from build123d import *

# Parameters (mm, degrees)
SKETCH1_W           = 39.4
SKETCH1_H           = 16.4
SKETCH1_R           = 1.725
BOSS_EXTRUDE1_DEPTH = 1.2
SKETCH2_W           = 12.5
SKETCH2_H           = 4
SKETCH2_W_2         = 4
SKETCH2_H_2         = 10.5
BOSS_EXTRUDE2_DEPTH = 2.5
SKETCH3_W           = 11.3
SKETCH3_H           = 12.5
SKETCH3_W_2         = 12.75
SKETCH3_H_2         = 6.6
BOSS_EXTRUDE3_DEPTH = 6
BOSS_EXTRUDE4_DEPTH = 2


with BuildPart() as part:
    # Sketch1 → Boss-Extrude1 (new body)
    with BuildSketch(Plane(origin=(0, 0, 0), x_dir=(1, 0, 0), z_dir=(0, 1, 0))):
        Rectangle(SKETCH1_W, SKETCH1_H)
        with Locations(Location((-16.7, 5.2, 0), (0, 0, 270))):
            Circle(SKETCH1_R, mode=Mode.SUBTRACT)
        with Locations(Location((2.3, 5.2, 0), (0, 0, 270))):
            Circle(SKETCH1_R, mode=Mode.SUBTRACT)
    extrude(amount=BOSS_EXTRUDE1_DEPTH)

    # Sketch2 → Boss-Extrude2 (add)
    with BuildSketch(Plane(origin=(0, 1.2, 0), x_dir=(1, 0, 0), z_dir=(0, 1, 0))):
        with Locations((-7.45, -1.2)):
            Rectangle(SKETCH2_W, SKETCH2_H)
        with Locations((8.2, -0.05)):
            Rectangle(SKETCH2_W_2, SKETCH2_H_2)
    extrude(amount=BOSS_EXTRUDE2_DEPTH)

    # Sketch3 → Boss-Extrude3 (add)
    with BuildSketch(Plane.XZ):
        with Locations((14.05, 0)):
            Rectangle(SKETCH3_W, SKETCH3_H)
        with Locations((-7.2, -4.9)):
            Rectangle(SKETCH3_W_2, SKETCH3_H_2)
    extrude(amount=BOSS_EXTRUDE3_DEPTH)

    # Sketch4 → Boss-Extrude4 (add, symmetric)
    with BuildSketch(Plane(origin=(0, -3, 0), x_dir=(-1, 0, 0), z_dir=(0, -1, 0))):
        with BuildLine():
            Line((1.825, 8.2), (13.224013115, 11.95))
            ThreePointArc((13.224013115, 11.95), (14.96605462, 13.598761551), (16.825, 12.083028945))
            Line((16.825, 12.083028945), (16.627742085, 12.050024171))
            ThreePointArc((16.627742085, 12.050024171), (14.909005352, 13.395228648), (13.416459603, 11.802765704))
            Line((13.416459603, 11.802765704), (2.465, 8.2))
            Line((2.465, 8.2), (1.825, 8.2))
        make_face()
    extrude(amount=BOSS_EXTRUDE4_DEPTH, both=True)


solid = part.part
Read the model definition and answer for the solid it produces. Units are mm, in the model's axes. A direction names the side the tool comes from. Coordinates: 2 decimals unless noted, no trailing zeros. Order: outer loops, then holes, each group sorted by start corner. A loop starts at its lowest first (then second) coordinate and runs counter-clockwise, first axis right, second up. Notation, with made-up numbers: (3, 80) -> (35, 80) arc R16 ccw to (35, 89) -> close; hole circle Ø5 at (6.5, 6). An arc over 180 degrees is marked (long way). Answer as a JSON object with one key per item and string values.
1) A tool of negligible diameter and unlimited length cuts with its end or side. For faces 1 (the face through (-8.017, -3.028, -10.027)), 2 (the face through (6.2, 2, 0)), 3 (the face through (-7, -3, -1.6)), 4 (the face through (-13.7, 2, 1)), 5 (the face through (8, 2, 5.3)), from which of +Z, -Z, +X, -X, +Y, -Y can it reach the whole face along a straight path? Write none if from no direction.
Model answer:
{"face 1": "-X, +Y, -Y", "face 2": "+Z, -Z, +Y", "face 3": "+Z, -X, -Y", "face 4": "+Z, -Z, -X, +Y", "face 5": "+Z, +X, -X, +Y"}
2) The mould has two halves that part along Z. Classify faces 6 (the face through (14, -3, -6.25)), 7 (the face through (3.47, 0.59, -6.47)), 8 (the face through (14, -3, 6.25)): released by +Z, released by -Z, zero draft, split by the parting line, or undercut.
Model answer:
{"face 6": "released by -Z", "face 7": "undercut", "face 8": "released by +Z"}
3) A cutting plane is placed at A-A, the plane y = 1.75. Determine the outline of the cut face in (x, z), plus the area to 3 significant figures.
Model answer:
{"outline": "(-13.7, -0.8) -> (-1.2, -0.8) -> (-1.2, 3.2) -> (-13.7, 3.2) -> close; (6.2, -5.2) -> (10.2, -5.2) -> (10.2, 5.3) -> (6.2, 5.3) -> close", "area": "92.0 mm²"}
4) Each of these flat-tipped pins is pushed along its axis until it touches: pin 1 (1.2 mm diameter, centred on x = 7.5, y = 2, fed in from +Z); pin 2 (1.2 mm diameter, centred on x = 7.5, y = 2, fed in from -Z); pin 3 (1.5 mm diameter, centred on x = 9.5, y = -2.5, fed in from +Z). Where does it stop, or does it pass through?
Model answer:
{"pin 1": "stops at z = 5.3", "pin 2": "stops at z = -5.2", "pin 3": "stops at z = 6.25"}
5) A cutting plane is placed at B-B, the plane x = 2.3. Determine the outline of the cut face in (y, z) (3 decimals), plus the area to 3 significant figures.
Model answer:
{"outline": "(0, -8.2) -> (1.2, -8.2) -> (1.2, -6.925) -> (0, -6.925) -> close; (0, -3.475) -> (1.2, -3.475) -> (1.2, 8.2) -> (0, 8.2) -> close", "area": "15.5 mm²"}
6) Consider line 1 along X through (y, z) = (0.5, -5.2) (3 decimals); line 2 along Y through (x, z) = (-2.5, 0.5); line 3 along X through (y, z) = (-3.75, -4.5) (3 decimals). Determine where each line is inside the solid, lowest interval first. Write a range as from..to.
Model answer:
{"line 1": "x = -19.7..-18.425, -14.975..0.575, 4.025..19.7", "line 2": "y = 0..3.7", "line 3": "x = -13.575..-0.825, 8.4..19.7"}
7) A cutting plane is placed at D-D, the plane z = 0.75. Determine the outline of the cut face in (x, y), plus the area to 3 significant figures.
Model answer:
{"outline": "(-19.7, 0) -> (8.4, 0) -> (8.4, -6) -> (19.7, -6) -> (19.7, 1.2) -> (10.2, 1.2) -> (10.2, 3.7) -> (6.2, 3.7) -> (6.2, 1.2) -> (-1.2, 1.2) -> (-1.2, 3.7) -> (-13.7, 3.7) -> (-13.7, 1.2) -> (-19.7, 1.2) -> close", "area": "156 mm²"}
8) A cutting plane is placed at C-C, the plane z = -4.5. Determine the outline of the cut face in (x, y) (3 decimals).
Model answer:
{"outline": "(-19.7, 0) -> (-18.277, 0) -> (-18.277, 1.2) -> (-19.7, 1.2) -> close; (-15.123, 0) -> (-13.575, 0) -> (-13.575, -6) -> (-0.825, -6) -> (-0.825, 0) -> (0.723, 0) -> (0.723, 1.2) -> (-15.123, 1.2) -> close; (3.877, 0) -> (8.4, 0) -> (8.4, -6) -> (19.7, -6) -> (19.7, 1.2) -> (10.2, 1.2) -> (10.2, 3.7) -> (6.2, 3.7) -> (6.2, 1.2) -> (3.877, 1.2) -> close"}
